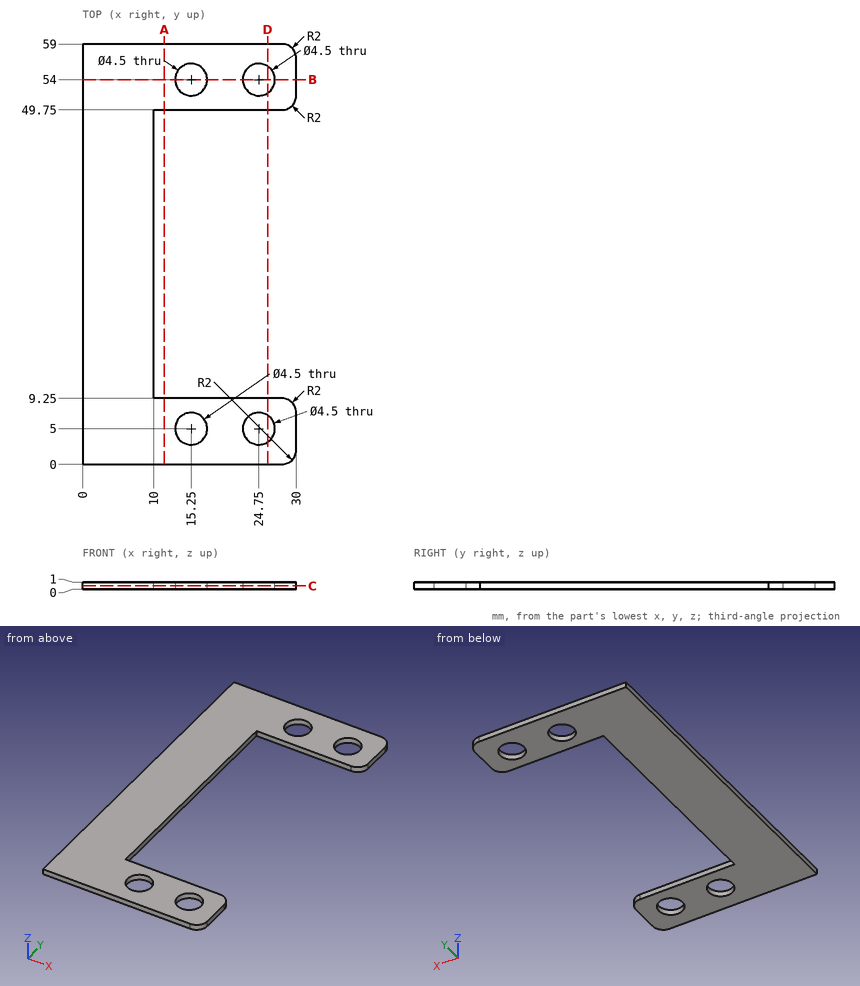
Input: dimensioned drawing with shaded views. Units: mm. Origin: part minimum x, y, z. Coordinates: 2 decimals unless noted, no trailing zeros. Loops run counter-clockwise (first coordinate to the right, second up) from the corner with the lowest first, then second, coordinate; pieces in that order, holes last.
Q1. Line query: line 1 along Y through (x, z) = (15.25, 0.3); line 2 along Y through (x, z) = (28, 0.65); line 3 along Y through (x, z) = (26.5, 0.3). Output: solid intervals per line, ascending.
Results are:
line 1: y = 0 to 2.75, 7.25 to 9.25, 49.75 to 51.75, 56.25 to 59
line 2: y = 0 to 9.25, 49.75 to 59
line 3: y = 0 to 3.59, 6.41 to 9.25, 49.75 to 52.59, 55.41 to 59
Q2. Section D-D, the plane x = 26. Return the cut outline in (y, z).
Results are:
outline: (0, 0) - (3.13, 0) - (3.13, 1) - (0, 1) - close; (6.87, 0) - (9.25, 0) - (9.25, 1) - (6.87, 1) - close; (49.75, 0) - (52.13, 0) - (52.13, 1) - (49.75, 1) - close; (55.87, 0) - (59, 0) - (59, 1) - (55.87, 1) - close
Q3. Section B-B, the plane y = 54. Return the cut outline in (x, z).
Results are:
outline: (0, 0) - (13, 0) - (13, 1) - (0, 1) - close; (17.5, 0) - (22.5, 0) - (22.5, 1) - (17.5, 1) - close; (27, 0) - (30, 0) - (30, 1) - (27, 1) - close
Q4. Section A-A, the plane x = 11.5. Return the cut outline in (y, z), and give its area (3 significant figures).
Results are:
outline: (0, 0) - (9.25, 0) - (9.25, 1) - (0, 1) - close; (49.75, 0) - (59, 0) - (59, 1) - (49.75, 1) - close
area: 18.5 mm2
Q5. Section C-C, the plane z = 0.5. Return the cut outline in (x, y).
Results are:
outline: (0, 0) - (28, 0) arc R2 ccw to (30, 2) - (30, 7.25) arc R2 ccw to (28, 9.25) - (10, 9.25) - (10, 49.75) - (28, 49.75) arc R2 ccw to (30, 51.75) - (30, 57) arc R2 ccw to (28, 59) - (0, 59) - close; hole circle Ø4.5 at (15.25, 5); hole circle Ø4.5 at (15.25, 54); hole circle Ø4.5 at (24.75, 5); hole circle Ø4.5 at (24.75, 54)
Q6. Contact query for flat-ended pins moving along their axis: pin 1 (5 mm diameter, centred on x = 24.75, y = 54, fed in from +Z); pin 2 (5 mm diameter, centred on x = 27, y = 13.5, fed in from -Z). Output: stop coordinate, or through.
Results are:
pin 1: stops at z = 1
pin 2: passes through
